```python
from build123d import *

# Parameters (mm, degrees)
SKETCH_1_W          = 25
SKETCH_1_H          = 25
EXTRUDE_1_DEPTH     = 90
EXTRUDE_START       = 33
SKETCH_1_3_R        = 6
SKETCH_1_3_W        = 25
SKETCH_1_3_H        = 25
EXTRUDE_2_DEPTH     = 10
SKETCH_3_W          = 12
SKETCH_3_H          = 15
SKETCH_3_W_2        = 10
SKETCH_3_H_2        = 4
CUT_EXTRUDE_3_DEPTH = 114.798066767


with BuildPart() as part:
    # Эскиз1 → Бобышка-Вытянуть1 (new body)
    with BuildSketch(Plane.XY):
        Rectangle(SKETCH_1_W, SKETCH_1_H)
    extrude(amount=EXTRUDE_1_DEPTH)

    # Эскиз1<3> → Бобышка-Вытянуть2 (add)
    with BuildSketch(Plane.XY.offset(EXTRUDE_START)):
        with BuildLine():
            Line((-21.650635095, 12.5), (-40, 12.5))
            ThreePointArc((-40, 12.5), (-52.5, 0), (-40, -12.5))
            Line((-40, -12.5), (-21.650635095, -12.5))
            ThreePointArc((-21.650635095, -12.5), (0, -25), (21.650635095, -12.5))
            Line((21.650635095, -12.5), (40, -12.5))
            Line((40, -12.5), (40, -6))
            ThreePointArc((40, -6), (34, 0), (40, 6))
            Line((40, 6), (40, 12.5))
            Line((40, 12.5), (21.650635095, 12.5))
            ThreePointArc((21.650635095, 12.5), (0, 25), (-21.650635095, 12.5))
        make_face()
        with Locations((-40, 0)):
            Circle(SKETCH_1_3_R, mode=Mode.SUBTRACT)
        Rectangle(SKETCH_1_3_W, SKETCH_1_3_H, mode=Mode.SUBTRACT)
    extrude(amount=EXTRUDE_2_DEPTH)

    # Эскиз3 → Вырез-Вытянуть3 (cut, through all)
    with BuildSketch(Plane.ZY.offset(-12.5)):
        with Locations((74, 0)):
            Rectangle(SKETCH_3_W, SKETCH_3_H)
        with Locations((85, 0)):
            Rectangle(SKETCH_3_W_2, SKETCH_3_H_2)
    extrude(amount=CUT_EXTRUDE_3_DEPTH, mode=Mode.SUBTRACT)


solid = part.part
```
Could you check a few things on this model? Use its own coordinates, in mm. A direction names the side the tool comes from. Round coordinates to 2 decimals unless told otherwise and drop trailing zeros. Loops run counter-clockwise (first coordinate to the right, second up) from the corner with the lowest first, then second, coordinate; pieces in that order, holes last. Notation, with made-up numbers: (39.5, -32) - (98.5, -32) arc R13 cw to (98.5, -12) - close; hole circle Ø1 at (40.5, 63.25). An arc over 180 degrees is marked (long way). Use CSV: the item, a comma, the result in double quotes.
Item 1: If we section it at C-C on x = -36: List the corners of the cut face in (y, z) for me.
Here are the results:
outline,"(-12.5, 33) - (-4.47, 33) - (-4.47, 43) - (-12.5, 43) - close; (4.47, 33) - (12.5, 33) - (12.5, 43) - (4.47, 43) - close"
Item 2: For faces 4 (the flat face through (0, -5, 80)), 5 (the flat face through (-12.5, 0, 66)), 6 (the flat face through (12.5, 0, 66)), 7 (the flat face through (-31, -12.5, 38)), which set-ups out of +Z, -Z, +X, -X, +Y, -Y let a thin tool reach every point of the face, with its end or its side?
Here are the results:
face 4,"+X, -X"
face 5,"+Z, -X, +Y, -Y"
face 6,"+Z, +X, +Y, -Y"
face 7,"+Z, -Z, -X, -Y"
Item 3: If we mould it in two halves opening along Z, with no side actions, what happens to faces 1 (the cylindrical face through (34, 0, 38)), 2 (the flat face through (0, 5, 80)), 3 (the flat face through (0, 0, 0))? For each: pulls with the +Z half, pulls with the -Z half, needs draft (parallel to the pull), parting line crosses it, or undercut.
Here are the results:
face 1,"needs draft"
face 2,"undercut"
face 3,"pulls with the -Z half"
Item 4: Will these pins go through, and if not, where does the flat tip stop? pin 1 (12 mm diameter, centred on x = 3.5, z = 79, fed in from +Y); pin 2 (12 mm diameter, centred on y = 5, z = 37.5, fed in from +X); pin 3 (3 mm diameter, centred on x = 4, z = 85.5, fed in from -Y); pin 4 (3 mm diameter, centred on y = -12, z = 61, fed in from +X).
Here are the results:
pin 1,"stops at y = 12.5"
pin 2,"stops at x = 40"
pin 3,"stops at y = -12.5"
pin 4,"stops at x = 12.5"
Item 5: If we section it at D-D on y = 10.5: List the corners of the cut face in (x, z) for me.
Here are the results:
outline,"(-46.78, 33) - (-12.5, 33) - (-12.5, 0) - (12.5, 0) - (12.5, 33) - (40, 33) - (40, 43) - (12.5, 43) - (12.5, 90) - (-12.5, 90) - (-12.5, 43) - (-46.78, 43) - close"
Item 6: If we section it at A-A on z = 77: List the corners of the cut face in (x, y) for me, then the cut area to 3 significant figures.
Here are the results:
outline,"(-12.5, -12.5) - (12.5, -12.5) - (12.5, -7.5) - (-12.5, -7.5) - close; (-12.5, 7.5) - (12.5, 7.5) - (12.5, 12.5) - (-12.5, 12.5) - close"
area,"250 mm²"
Item 7: I need wall thicknesses on L1, parallel to Z at x = -5, y = -3.5; L2, parallel to Y at x = 1, z = 85; L3, parallel to Y at x = -40, z = 39.5. Which ranges of each line are inside material? Lowest first, please. Write a range as [from, to].
Here are the results:
L1,"z = [0, 68], [80, 90]"
L2,"y = [-12.5, -2], [2, 12.5]"
L3,"y = [-12.5, -6], [6, 12.5]"
Item 8: If we section it at B-B on y = 0: List the corners of the cut face in (x, z) for me, then the cut area to 4 significant figures.
Here are the results:
outline,"(-52.5, 33) - (-46, 33) - (-46, 43) - (-52.5, 43) - close; (-34, 33) - (-12.5, 33) - (-12.5, 0) - (12.5, 0) - (12.5, 33) - (34, 33) - (34, 43) - (12.5, 43) - (12.5, 68) - (-12.5, 68) - (-12.5, 43) - (-34, 43) - close"
area,"2,195 mm²"
